Read the model definition and answer for the solid it produces. Units are mm, in the model's axes. Face numbers are marked on the shaded views. Give positions to 0.01 mm unless a question says otherwise; leave off trailing zeros. Loops run counter-clockwise (first coordinate to the right, second up) from the corner with the lowest first, then second, coordinate; pieces in that order, holes last. Notation, with made-up numbers: (48, -20) - (98, -20) arc R17 cw to (98, -14) - close; hole circle Ø4 at (-26.5, 31). An arc over 180 degrees is marked (long way). Write each question's results on one line, items separated by ' | '. Start each with the question number.
Q1. The part is cut by section C-C, the plane z = 11. Write down the section's boundary in (x, y).
Q2. The part is cut by section B-B, the plane y = -0.3. Write down the section's boundary in (x, z).
Q3. Determine the mould class of the marked faces 1, 2 and 3 for opening direction Y: +Y half, -Y half, draft (parallel to the pull), parting line (faces both ways), or undercut.
Q4. Find the intervals of material crossed by line 1 (Y direction, x = 2.6, z = 15); line 2 (Z direction, x = 1.1, y = -0.95); line 3 (Y direction, x = 0.15, z = 5), in increasing order. Write a range as from..to.
Q5. Given pin 1 (2 mm diameter, centred on x = 2.5, z = 22.5, fed in from -Y), flat-ended and moving along its own axis, determine where the tip first touches the part or whether it passes through.
Q6. The part is cut by section A-A, the plane x = 0. Write down the section's boundary in (y, z).
Q7. The part is cut by section D-D, the plane y = -2.4. Write down the section's boundary in (x, z), plus the area to 3 significant figures.
```python
from build123d import *

# Parameters (mm, degrees)
S01_M6_CONNECTING_STUD_R      = 3
F_01_M6_CONNECTING_STUD_DEPTH = 30
F_02_START                    = -0.1
F_02_HEX_KEY_SOCKET_DEPTH     = 3.1


with BuildPart() as part:
    # S01 - M6 connecting stud → 01 - M6 connecting stud (new body)
    with BuildSketch(Plane.XY):
        Circle(S01_M6_CONNECTING_STUD_R)
    extrude(amount=F_01_M6_CONNECTING_STUD_DEPTH)

    # S02 - Hex key socket → 02 - Hex key socket (cut)
    with BuildSketch(Plane.XY.offset(F_02_START)):
        Polygon((1.732050808, 0), (0.866025404, 1.5), (-0.866025404, 1.5), (-1.732050808, 0), (-0.866025404, -1.5), (0.866025404, -1.5), align=None)
    extrude(amount=F_02_HEX_KEY_SOCKET_DEPTH, mode=Mode.SUBTRACT)


solid = part.part
```
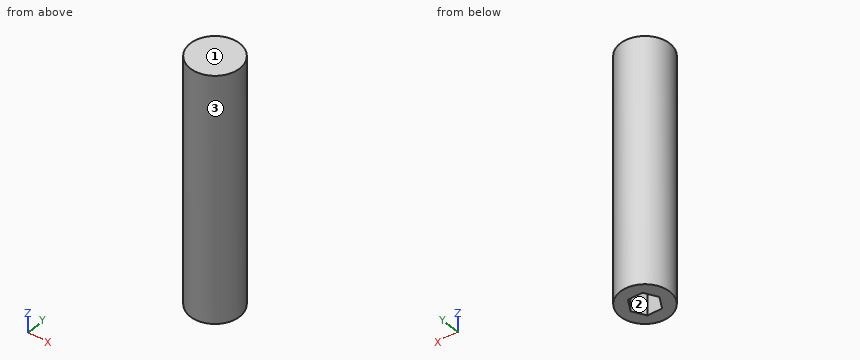
Check sheet entries:
1) outline: circle Ø6 at (0, 0)
2) outline: (-2.98, 0) - (-1.56, 0) - (-1.56, 3) - (1.56, 3) - (1.56, 0) - (2.98, 0) - (2.98, 30) - (-2.98, 30) - close
3) face 1: draft | face 2: undercut | face 3: parting line
4) line 1: y = -1.5..1.5 | line 2: z = 3..30 | line 3: y = -3..3
5) pin 1: stops at y = -2.6
6) outline: (-3, 0) - (-1.5, 0) - (-1.5, 3) - (1.5, 3) - (1.5, 0) - (3, 0) - (3, 30) - (-3, 30) - close
7) outline: (-1.8, 0) - (1.8, 0) - (1.8, 30) - (-1.8, 30) - close | area: 108 mm^2
